```python
from build123d import *

# Parameters (mm, degrees)
F0_R     = 30.15
F1_DEPTH = 18
F2_R     = 24.61
F3_DEPTH = 6
F4_R     = 5.99999
F5_R     = 14.5
F6_DEPTH = 25


# Not quite as in the source:
# - a fillet or chamfer is up to 0.001 mm smaller than in the source, because OpenCascade refuses the exact size


with BuildPart() as f1:
    # F0 (on Front) → F1 (new body)
    with BuildSketch(Plane.XZ):
        Circle(F0_R)
    extrude(amount=F1_DEPTH)

    # F2 (on face) → F3 (cut)
    with BuildSketch(Plane.XZ.offset(18)):
        Circle(F2_R)
    extrude(amount=-F3_DEPTH, mode=Mode.SUBTRACT)

    # F4 (radius 6 in the source; OpenCascade refuses exactly that, so slightly less here)
    f4_edges = [f1.edges().sort_by_distance(p)[0] for p in [
        (-24.61, -12, 0),
    ]]
    fillet(f4_edges, radius=F4_R)

    # F5 (on face) → F6 (cut)
    with BuildSketch(Plane.XZ.offset(12)):
        Circle(F5_R)
    extrude(amount=-F6_DEPTH, mode=Mode.SUBTRACT)

    # F7 (on Top) → F8 (revolve, cut)
    with BuildSketch(Plane.XY):
        Polygon((-30.15, -18), (-25.6668464834, -18), (-30.15, -14.5470285541), align=None)
    revolve(axis=Axis((0, -2.2485724185, 0), (0, -1, 0)), mode=Mode.SUBTRACT)


solid = f1.part
```
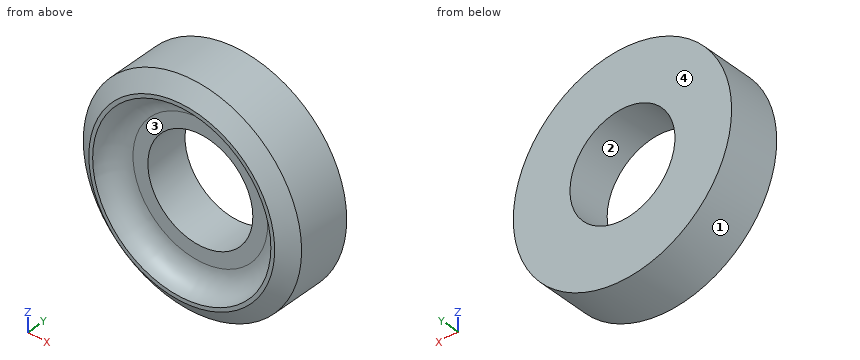
For this review, take the finished solid that the model builds, in its own axes (mm). Face numbers are marked on the shaded views. Coordinates: 2 decimals unless noted, no trailing zeros. Loops run counter-clockwise (first coordinate to the right, second up) from the corner with the lowest first, then second, coordinate; pieces in that order, holes last.
1. Mouldability with a two-part tool opening along X and no side actions: class the marked faces 1, 2, 3 and 4 as +X half, -X half, draft (parallel to the pull), parting line (faces both ways), or undercut.
2. Add section C-C, the plane y = -11. Give the boundary of the cut face in (x, z), then the cut area to 3 significant figures.
3. Insertion check: P1, Ø4, axis at y = -13, z = 17.5, coming from the +X side; P2, Ø10, axis at x = 20, y = -11, coming from the -Z side; P3, Ø1, axis at x = 22.5, y = -9.5, coming from the +Z side. Each pin has a flat end and moves straight along its axis. Give the tip position at first contact, or say it passes through.
4. For line 1 (Z direction, x = 0, y = -9); line 2 (Z direction, x = 13, y = -6); line 3 (X direction, y = -13.25, z = -7), list the stretches that pass through material, from the lowest coordinate up.
Result:
1. face 1: parting line
1. face 2: undercut
1. face 3: undercut
1. face 4: draft
2. outline: circle Ø60.3 at (0, 0); hole circle Ø29 at (0, 0)
2. area: 2,200 mm2
3. P1: stops at x = 25.86
3. P2: stops at z = -26.15
3. P3: stops at z = 20.62
4. line 1: z = -30.15 to -14.5, 14.5 to 30.15
4. line 2: z = -27.2 to -6.42, 6.42 to 27.2
4. line 3: x = -29.33 to -21.15, 21.15 to 29.33
